```python
from build123d import *

# Parameters (mm, degrees)
SKETCH1_R                    = 6.49
SKETCH1_R_2                  = 1
BOSS_EXTRUDE1_DEPTH          = 1
BOSS_EXTRUDE2_START          = -1.2
SKETCH1_3_R                  = 6.49
SKETCH1_3_R_2                = 1
BOSS_EXTRUDE2_DEPTH          = 1.2
BOSS_EXTRUDE3_START          = 1
SKETCH2_R                    = 6.49
SKETCH2_R_2                  = 1
BOSS_EXTRUDE3_DEPTH          = 1
SKETCH3_R                    = 7.49
BOSS_EXTRUDE4_DEPTH          = 20
F_7_0_7_DIAMETER_HOLE1_D     = 7
F_7_0_7_DIAMETER_HOLE1_DEPTH = 16.7
F_2_0MM_DOWEL_HOLE1_D        = 2
F_2_0MM_DOWEL_HOLE1_DEPTH    = 4
F_2_0MM_DOWEL_HOLE1_TIP      = 0.600860619
FILLET1_R                    = 2
F_4_5_4_5_DIAMETER_HOLE2_D   = 4.5
CUT_EXTRUDE2_REACH           = 31.073
CUT_EXTRUDE2_END_RADIUS      = 3.5
SKETCH10_R                   = 2.25
CUT_EXTRUDE2_DRAFT           = -7


with BuildPart() as part:
    # Sketch1 → Boss-Extrude1 (new body)
    # profile 1 of 2: a face of its own
    with BuildSketch(Plane.XY):
        Circle(SKETCH1_R)
        with Locations((0, 4.5)):
            Circle(SKETCH1_R_2, mode=Mode.SUBTRACT)
    # profile 2 of 2: a face of its own
    with BuildSketch(Plane.XY):
        with Locations((0, 4.5)):
            Circle(SKETCH1_R_2)
    extrude(amount=BOSS_EXTRUDE1_DEPTH)

    # Sketch1_3 → Boss-Extrude2 (add)
    # profile 1 of 3: a face of its own
    with BuildSketch(Plane.XY.offset(BOSS_EXTRUDE2_START)):
        with BuildLine():
            ThreePointArc((-7.29, -5.260798418), (-4.094235107, -8.003582878), (0, -8.99))
            ThreePointArc((0, -8.99), (4.094235107, -8.003582878), (7.29, -5.260798418))
            Line((7.29, -5.260798418), (7.29, 5.260798418))
            ThreePointArc((7.29, 5.260798418), (4.094235107, 8.003582878), (0, 8.99))
            ThreePointArc((0, 8.99), (-4.094235107, 8.003582878), (-7.29, 5.260798418))
            Line((-7.29, 5.260798418), (-7.29, -5.260798418))
        make_face()
        Circle(SKETCH1_3_R, mode=Mode.SUBTRACT)
    # profile 2 of 3: a face of its own
    with BuildSketch(Plane.XY.offset(BOSS_EXTRUDE2_START)):
        Circle(SKETCH1_3_R)
        with Locations((0, 4.5)):
            Circle(SKETCH1_3_R_2, mode=Mode.SUBTRACT)
    # profile 3 of 3: a face of its own
    with BuildSketch(Plane.XY.offset(BOSS_EXTRUDE2_START)):
        with Locations((0, 4.5)):
            Circle(SKETCH1_3_R_2)
    extrude(amount=BOSS_EXTRUDE2_DEPTH)

    # Sketch2 → Boss-Extrude3 (add)
    # profile 1 of 5: a face of its own
    with BuildSketch(Plane(origin=(0, 0, -1.2), x_dir=(-1, 0, 0), z_dir=(0, 0, -1)).offset(BOSS_EXTRUDE3_START)):
        with BuildLine():
            ThreePointArc((7.29, 5.260798418), (0, 8.99), (-7.29, 5.260798418))
            Line((-7.29, 5.260798418), (-7.29, -5.260798418))
            ThreePointArc((-7.29, -5.260798418), (0, -8.99), (7.29, -5.260798418))
            Line((7.29, -5.260798418), (7.29, 5.260798418))
        make_face()
        with Locations(Location((0, 0, 0), (0, 0, 180))):
            Circle(SKETCH2_R, mode=Mode.SUBTRACT)
    # profile 2 of 5: a face of its own
    with BuildSketch(Plane(origin=(0, 0, -1.2), x_dir=(-1, 0, 0), z_dir=(0, 0, -1)).offset(BOSS_EXTRUDE3_START)):
        with Locations(Location((0, 0, 0), (0, 0, 180))):
            Circle(SKETCH2_R)
        with Locations((0, 4.5)):
            Circle(SKETCH2_R_2, mode=Mode.SUBTRACT)
    # profile 3 of 5: a face of its own
    with BuildSketch(Plane(origin=(0, 0, -1.2), x_dir=(-1, 0, 0), z_dir=(0, 0, -1)).offset(BOSS_EXTRUDE3_START)):
        with BuildLine():
            ThreePointArc((-7.29, 5.260798418), (-8.99, 0), (-7.29, -5.260798418))
            Line((-7.29, -5.260798418), (-7.29, 5.260798418))
        make_face()
    # profile 4 of 5: a face of its own
    with BuildSketch(Plane(origin=(0, 0, -1.2), x_dir=(-1, 0, 0), z_dir=(0, 0, -1)).offset(BOSS_EXTRUDE3_START)):
        with BuildLine():
            Line((7.29, 5.260798418), (7.29, -5.260798418))
            ThreePointArc((7.29, -5.260798418), (8.554449135, -2.764326319), (8.99, 0))
            ThreePointArc((8.99, 0), (8.554449135, 2.764326319), (7.29, 5.260798418))
        make_face()
    # profile 5 of 5: a face of its own
    with BuildSketch(Plane(origin=(0, 0, -1.2), x_dir=(-1, 0, 0), z_dir=(0, 0, -1)).offset(BOSS_EXTRUDE3_START)):
        with Locations((0, 4.5)):
            Circle(SKETCH2_R_2)
    extrude(amount=-BOSS_EXTRUDE3_DEPTH)

    # Sketch3 → Boss-Extrude4 (add)
    with BuildSketch(Plane(origin=(0, 0, -2.2), x_dir=(-1, 0, 0), z_dir=(0, 0, -1))):
        Circle(SKETCH3_R)
    extrude(amount=BOSS_EXTRUDE4_DEPTH)

    # 7.0 _7_ Diameter Hole1
    with Locations(Plane(origin=(0, 0, -22.2), x_dir=(-1, 0, 0), z_dir=(0, 0, -1))):
        with Locations((0, 0)):
            Hole(F_7_0_7_DIAMETER_HOLE1_D / 2, depth=F_7_0_7_DIAMETER_HOLE1_DEPTH)

    # 2.0mm Dowel Hole1
    with Locations(Plane.XY.offset(1)):
        with Locations((0, 4.5)):
            Hole(F_2_0MM_DOWEL_HOLE1_D / 2, depth=F_2_0MM_DOWEL_HOLE1_DEPTH)
            with Locations((0, 0, -(F_2_0MM_DOWEL_HOLE1_DEPTH + F_2_0MM_DOWEL_HOLE1_TIP / 2))):  # 118° drill point
                Cone(0, F_2_0MM_DOWEL_HOLE1_D / 2, F_2_0MM_DOWEL_HOLE1_TIP, mode=Mode.SUBTRACT)

    # Fillet1
    fillet1_edges = [part.edges().sort_by_distance(p)[0] for p in [
        (7.49, 0, -22.2),
    ]]
    fillet(fillet1_edges, radius=FILLET1_R)

    # 4.5 _4.5_ Diameter Hole2 (through all)
    with Locations(Plane.XY.offset(1)):
        with Locations((0, 0)):
            Hole(F_4_5_4_5_DIAMETER_HOLE2_D / 2)

    # Cut-Extrude2: up to this cylinder (the profile starts outside it)
    cut_extrude2_end = Plane(origin=(0, 0, -14.7), z_dir=(0, 0, -1)) * Cylinder(CUT_EXTRUDE2_END_RADIUS, 70.146, mode=Mode.PRIVATE)



with BuildPart() as cut_extrude2_long_prism_1:
    # Sketch10 → Cut-Extrude2 (the long prism of profile 1, to be tilted and cut off)
    with BuildSketch(Plane(origin=(7.49, 0, 0), x_dir=(0, 0, -1), z_dir=(1, 0, 0))):
        with Locations((14.7, 0)):
            Circle(SKETCH10_R)
    extrude(amount=-CUT_EXTRUDE2_REACH)
    cut_extrude2_tool1_sides = [cut_extrude2_long_prism_1.faces().sort_by_distance(p)[0] for p in [
        (-8.0465, 0, -12.45),
    ]]
    draft(cut_extrude2_tool1_sides, Plane(origin=(7.49, 0, 0), x_dir=(0, 0, -1), z_dir=(1, 0, 0)), CUT_EXTRUDE2_DRAFT)  # the draft: side faces tilted about the start plane


with BuildPart() as part_1:
    add(part.part)
    cut_extrude2_tool1 = cut_extrude2_long_prism_1.part - cut_extrude2_end
    add(cut_extrude2_tool1.solids().sort_by_distance((7.49, 0, -14.7))[0], mode=Mode.SUBTRACT)


solid = part_1.part
```
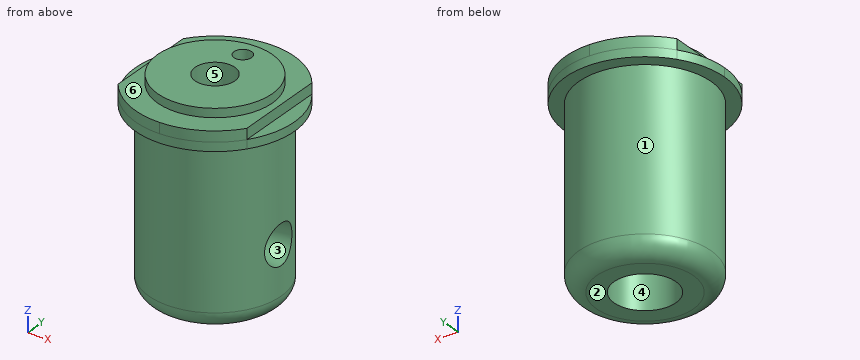
Design review of the part built by this model. Coordinates are the model's own, in mm. Face numbers are marked on the shaded views. A direction names the side the tool comes from. Round coordinates to 2 decimals unless told otherwise and drop trailing zeros. Write each loop counter-clockwise with the first axis right and the second up, starting at its lowest first coordinate (ties: lowest second). Pieces come first, ordered by that corner, then holes.
Item 1: For the marked faces 4, 5 and 6, list the 3-axis set-ups (+Z, -Z, +X, -X, +Y, -Y) from which the entire face can be reached by the end or side of a thin tool; tool diameter is ignored.
Item 2: For probe 1 along Y at (x, z) = (0, -2.75); probe 2 along Y at (x, z) = (0, -17); probe 3 along X at (y, z) = (4.5, -0.5), list the stretches that pass through material, from the lowest coordinate up.
Item 3: We need section B-B on z = -14.7. Write out the cut boundary in (x, y).
Item 4: We need section A-A on z = -9.75. Write out the cut boundary in (x, y).
Item 5: The part is to be moulded in two halves that separate along Y. For the marked faces 1, 2 and 3, say which applies: +Y half, -Y half, draft (parallel to the pull), parting line (faces both ways), or undercut.
Item 6: Clearance check with flat-ended pins moving along their axes: pin 1 Ø0.6 at (y, z) = (0, -0.5) entering from +X; pin 2 Ø6 at (y, z) = (2, -15) entering from +X; pin 3 Ø2.5 at (x, y) = (0, 0) entering from -Z; pin 4 Ø1.3 at (y, z) = (2.5, -0.5) entering from -X. State where each tip first meets the part, or that it passes through.
Returned:
1. face 4: -Z
1. face 5: +Z, -Z
1. face 6: +Z
2. probe 1: y = -7.49 to -2.25, 2.25 to 3.5, 5.5 to 7.49
2. probe 2: y = -7.49 to -3.5, 3.5 to 7.49
2. probe 3: x = -7.29 to -1, 1 to 7.29
3. outline: (3.06, -1.71) arc R3.5 cw (long way) to (3.06, 1.71) - (7.16, 2.21) arc R7.49 ccw (long way) to (7.16, -2.21) - close
4. outline: circle Ø14.98 at (0, 0); hole circle Ø7 at (0, 0)
5. face 1: parting line
5. face 2: draft
5. face 3: undercut
6. pin 1: stops at x = 7.29
6. pin 2: stops at x = 7.49
6. pin 3: passes through
6. pin 4: stops at x = -7.29
